Verification items for this drawing (mm, ordinates from the low corner). Coordinates: 2 decimals unless noted, no trailing zeros. Write each loop counter-clockwise with the first axis right and the second up, starting at its lowest first coordinate (ties: lowest second). Pieces come first, ordered by that corner, then holes. Notation, with made-up numbers: (-20, -30.75) -> (39, -30.75) arc R28 ccw to (39, 3.25) -> close; hole circle Ø4 at (33, 15). An arc over 180 degrees is marked (long way). One line per item, written item: value. Start each with the question number.
1) Scan lines: line 1 along Y through (x, z) = (5, 7.5) (1 decimal); line 2 along X through (y, z) = (13.75, 7.25) (1 decimal); line 3 along X through (y, z) = (7.25, 4) (1 decimal). Record each from-to range of solid material in increasing order. Write a range as [from, to].
2) Gauge pin test, flat ends, axial feed: P1, Ø6, axis at x = 2.5, z = 1.5, coming from the -Y side; P2, Ø1, axis at x = 5, y = 10.5, coming from the -Z side. Record the tip position at first contact, or that the pin passes through.
3) Draft check along X on the marked faces 1, 2, 3 and 4. Enter one of: +X half, -X half, draft (parallel to the pull), parting line (faces both ways), or undercut.
4) Sectioned sample at A-A on z = 6.75. Enter the section's corners in (x, y) (1 decimal).
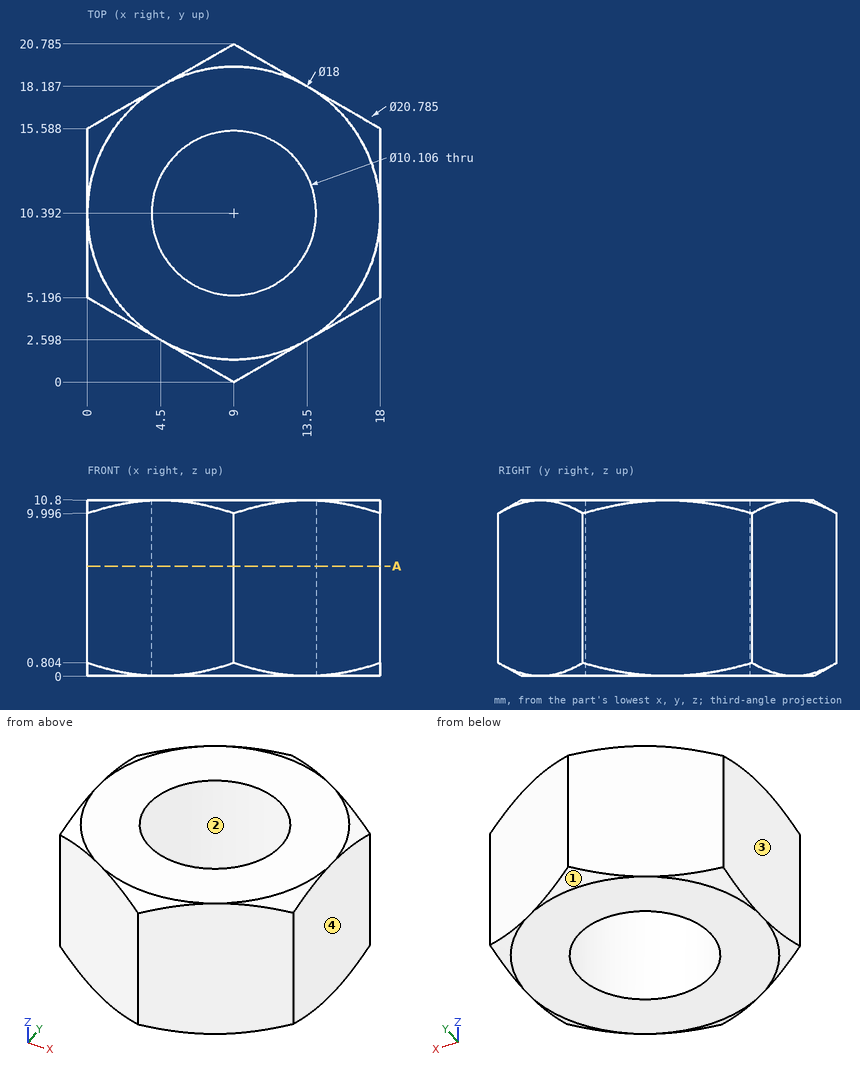
Answers:
1. line 1: y = [2.3, 7.3], [13.5, 18.5]
1. line 2: x = [0, 5.2], [12.8, 18]
1. line 3: x = [0, 5], [13, 18]
2. P1: stops at y = 2.02
2. P2: passes through
3. face 1: parting line
3. face 2: undercut
3. face 3: -X half
3. face 4: +X half
4. outline: (0, 5.2) -> (9, 0) -> (18, 5.2) -> (18, 15.6) -> (9, 20.8) -> (0, 15.6) -> close; hole circle Ø10.1 at (9, 10.4)
